Part print with two shaded views. Sizes in mm from the minimum x, y, z corner. Round coordinates to 2 decimals unless told otherwise and drop trailing zeros. Loops run counter-clockwise (first coordinate to the right, second up) from the corner with the lowest first, then second, coordinate; pieces in that order, holes last.
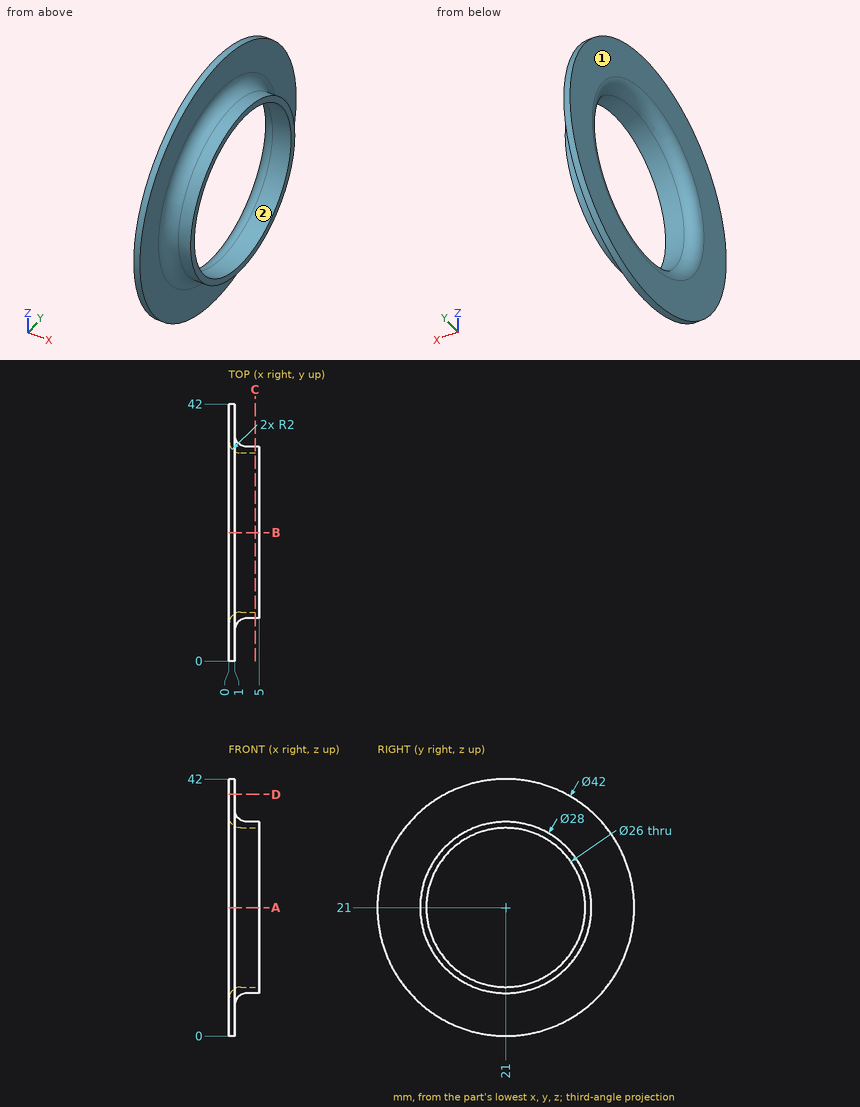
Item 1: Cut at C-C (x = 4.3). List the corners of the cut face in (y, z).
Verdict:
outline: circle Ø28 at (21, 21); hole circle Ø26 at (21, 21)
Item 2: Cut at D-D (z = 39.5). List the corners of the cut face in (x, y), plus the area to 3 significant figures.
Verdict:
outline: (0, 11.06) - (1, 11.06) - (1, 30.94) - (0, 30.94) - close
area: 19.9 mm2
Item 3: Wall check: L1, parallel to Z at x = 3.95, y = 21; L2, parallel to X at y = 4.5, z = 20; L3, parallel to Y at x = 3.6, z = 20. Give the ranges that are in metal, low to high.
Verdict:
L1: z = 7 to 8, 34 to 35
L2: x = 0 to 1
L3: y = 7.04 to 8.04, 33.96 to 34.96
Item 4: Cut at A-A (z = 21). List the corners of the cut face in (x, y), plus the area to 3 significant figures.
Verdict:
outline: (0, 0) - (1, 0) - (1, 5) arc R2 cw to (3, 7) - (5, 7) - (5, 8) - (2, 8) arc R2 ccw to (0, 6) - close; (0, 36) arc R2 ccw to (2, 34) - (5, 34) - (5, 35) - (3, 35) arc R2 cw to (1, 37) - (1, 42) - (0, 42) - close
area: 24.0 mm2
Item 5: Mould opens along Z. For the marked faces 1 and 2 say: released by +Z, released by -Z, zero draft, split by the parting line, or undercut.
Verdict:
face 1: zero draft
face 2: undercut
Item 6: Flat gauge pins, fed straight in: P1, Ø2, axis at x = 1, y = 18, coming from the +Z side; P2, Ø1, axis at x = 3.5, z = 11.5, coming from the +Y side; P3, Ø3, axis at x = 3.5, y = 35, coming from the +Z side. Where does each tip first touch, or does it go through?
Verdict:
P1: stops at z = 41.9
P2: stops at y = 31.72
P3: stops at z = 27.3
